Part print with two shaded views. Sizes in mm from the minimum x, y, z corner. A direction names the side the tool comes from. Round coordinates to 2 decimals unless told otherwise and drop trailing zeros. Loops run counter-clockwise (first coordinate to the right, second up) from the corner with the lowest first, then second, coordinate; pieces in that order, holes last. Notation, with made-up numbers: (87, 7.25) - (108, 7.25) arc R20 cw to (108, 29.25) - close; hole circle Ø2 at (88.5, -36.5). An arc over 180 degrees is marked (long way). Use a Markdown table: item, result.
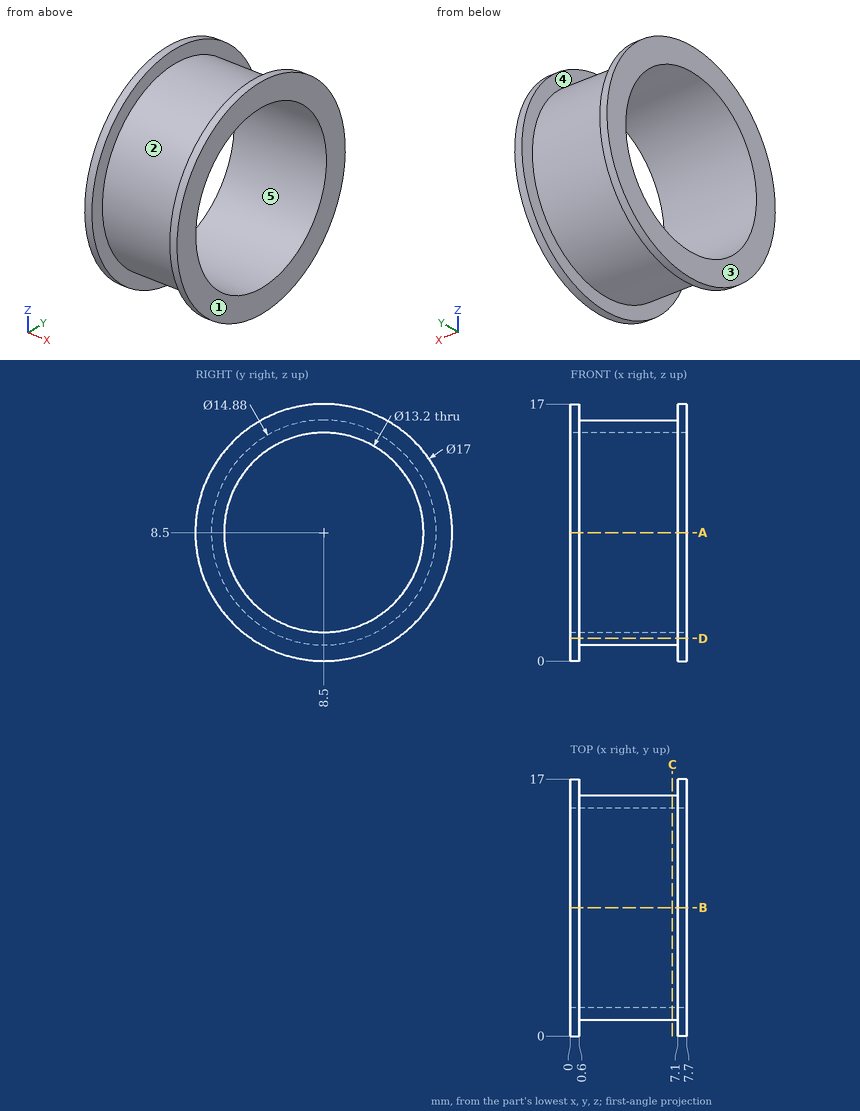
Q1. Probe line 1 (Y direction, x = 2.5, z = 8.5); line 2 (Y direction, x = 3.75, z = 4.5); line 3 (Z direction, x = 2.5, y = 3.5). List the from-to ranges inside material, lowest first.
Results found:
| item | result |
|---|---|
| line 1 | y = 1.06 to 1.9, 15.1 to 15.94 |
| line 2 | y = 2.23 to 3.25, 13.75 to 14.77 |
| line 3 | z = 2.99 to 4.19, 12.81 to 14.01 |
Q2. Which spindle directions (+Z, -Z, +X, -X, +Y, -Y) get a long thin tool onto all of the face, cutting with end or side? Do the marked faces 4 and 5. Say none if no direction does.
Results found:
| item | result |
|---|---|
| face 4 | none |
| face 5 | +X, -X |
Q3. Pull direction X, two halves, no side cores. Call the marked faces 1, 2 and 3: pulls with the +X half, pulls with the -X half, needs draft (parallel to the pull), parting line crosses it, or undercut.
Results found:
| item | result |
|---|---|
| face 1 | pulls with the +X half |
| face 2 | undercut |
| face 3 | pulls with the -X half |
Q4. Cut at C-C, the plane x = 6.75. List the corners of the cut face in (y, z).
Results found:
| item | result |
|---|---|
| outline | circle Ø14.88 at (8.5, 8.5); hole circle Ø13.2 at (8.5, 8.5) |
Q5. Cut at A-A, the plane z = 8.5. List the corners of the cut face in (x, y).
Results found:
| item | result |
|---|---|
| outline | (0, 0) - (0.6, 0) - (0.6, 1.06) - (7.1, 1.06) - (7.1, 0) - (7.7, 0) - (7.7, 1.9) - (0, 1.9) - close; (0, 15.1) - (7.7, 15.1) - (7.7, 17) - (7.1, 17) - (7.1, 15.94) - (0.6, 15.94) - (0.6, 17) - (0, 17) - close |
Q6. Cut at D-D, the plane z = 1.5. List the corners of the cut face in (x, y).
Results found:
| item | result |
|---|---|
| outline | (0, 3.68) - (0.6, 3.68) - (0.6, 5.98) - (7.1, 5.98) - (7.1, 3.68) - (7.7, 3.68) - (7.7, 13.32) - (7.1, 13.32) - (7.1, 11.02) - (0.6, 11.02) - (0.6, 13.32) - (0, 13.32) - close |
Q7. Drop flat-ended pins along their axis: pin 1 (2 mm diameter, centred on x = 4.5, y = 7.5, fed in from +Z); pin 2 (2 mm diameter, centred on x = 1.5, z = 6, fed in from +Y); pin 3 (4 mm diameter, centred on x = 6, y = 10.5, fed in from +Z). Give the stop position or say it passes through.
Results found:
| item | result |
|---|---|
| pin 1 | stops at z = 15.94 |
| pin 2 | stops at y = 16.75 |
| pin 3 | stops at z = 16.99 |
